Read the model definition and answer for the solid it produces. Units are mm, in the model's axes. Face numbers are marked on the shaded views. A direction names the side the tool comes from. Coordinates: 2 decimals unless noted, no trailing zeros. Order: outer loops, then holes, each group sorted by start corner. A loop starts at its lowest first (then second) coordinate and runs counter-clockwise, first axis right, second up. Notation, with made-up numbers: (-17.5, 41.25) -> (19.5, 41.25) arc R17 ccw to (19.5, 71.25) -> close; hole circle Ø4 at (35, -35). An arc over 180 degrees is marked (long way). Answer in a Markdown table with one row per item.
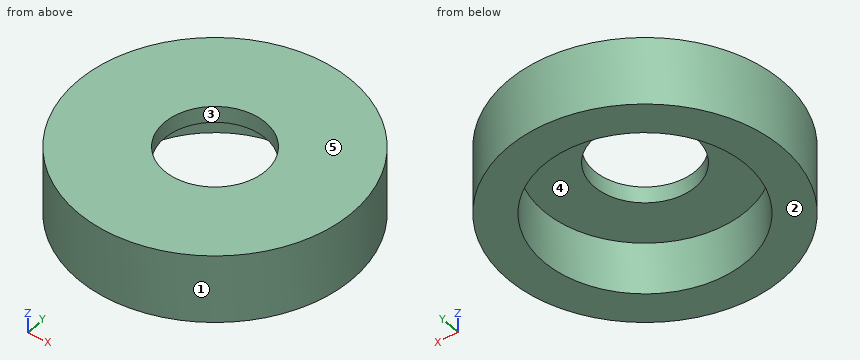
from build123d import *

# Parameters (mm, degrees)
SKETCH_1_R          = 42
EXTRUDE_1_DEPTH     = 21
SKETCH_2_R          = 31
CUT_EXTRUDE_2_DEPTH = 16
SKETCH_3_R          = 15.5
CUT_EXTRUDE_3_DEPTH = 62.514225997


with BuildPart() as part:
    # Эскиз1 → Вытянуть1 (new body)
    with BuildSketch(Plane.XY):
        with Locations(Location((0, 0, 0), (0, 0, 180))):
            Circle(SKETCH_1_R)
    extrude(amount=EXTRUDE_1_DEPTH)

    # Эскиз2 → Вытянуть2 (cut)
    with BuildSketch(Plane(origin=(0, 0, 0), x_dir=(-1, 0, 0), z_dir=(0, 0, -1))):
        Circle(SKETCH_2_R)
    extrude(amount=-CUT_EXTRUDE_2_DEPTH, mode=Mode.SUBTRACT)

    # Эскиз3 → Вытянуть3 (cut, through all)
    with BuildSketch(Plane(origin=(0, 0, 16), x_dir=(-1, 0, 0), z_dir=(0, 0, -1))):
        Circle(SKETCH_3_R)
    extrude(amount=-CUT_EXTRUDE_3_DEPTH, mode=Mode.SUBTRACT)


solid = part.part
Q1. The part is cut by section D-D (y = -17.5). Write down the section's boundary in (x, z).
Outcome:
| item | result |
|---|---|
| outline | (-38.18, 0) -> (-25.59, 0) -> (-25.59, 16) -> (25.59, 16) -> (25.59, 0) -> (38.18, 0) -> (38.18, 21) -> (-38.18, 21) -> close |
Q2. For the marked faces 4 and 5, determine the directions among +Z, -Z, +X, -X, +Y, -Y from which every point of the face is accessible in a straight line to the end or side of a thin tool.
Outcome:
| item | result |
|---|---|
| face 4 | -Z |
| face 5 | +Z, +X, -X, +Y, -Y |
Q3. The part is cut by section C-C (z = 6.75). Write down the section's boundary in (x, y), then the cut area to 3 significant figures.
Outcome:
| item | result |
|---|---|
| outline | circle Ø84 at (0, 0); hole circle Ø62 at (0, 0) |
| area | 2,520 mm² |
Q4. The part is cut by section A-A (x = 0). Write down the section's boundary in (y, z), then the cut area to 3 significant figures.
Outcome:
| item | result |
|---|---|
| outline | (-42, 0) -> (-31, 0) -> (-31, 16) -> (-15.5, 16) -> (-15.5, 21) -> (-42, 21) -> close; (15.5, 16) -> (31, 16) -> (31, 0) -> (42, 0) -> (42, 21) -> (15.5, 21) -> close |
| area | 617 mm² |
Q5. Consider line 1 (Y direction, x = 0, z = 3.5); line 2 (Y direction, x = 0, z = 18.65); line 3 (Z direction, x = 3, y = 28). Determine where each line is inside the solid, lowest interval first.
Outcome:
| item | result |
|---|---|
| line 1 | -42 to -31, 31 to 42 |
| line 2 | -42 to -15.5, 15.5 to 42 |
| line 3 | 16 to 21 |
Q6. For a pull along X with two mould halves and no side action, classify the marked faces 1, 2 and 3 as pulls with the +X half, pulls with the -X half, needs draft (parallel to the pull), parting line crosses it, or undercut.
Outcome:
| item | result |
|---|---|
| face 1 | parting line crosses it |
| face 2 | needs draft |
| face 3 | undercut |
Q7. Given pin 1 (4 mm diameter, centred on x = 16, z = 17, fed in from +Y); pin 2 (12 mm diameter, centred on x = 32.5, y = -7, fed in from -Z); pin 3 (6 mm diameter, centred on x = -32, z = 17.5, fed in from -Y); pin 4 (10 mm diameter, centred on x = -7, z = 11, fed in from +Y), each flat-ended and moving along its own axis, determine where each tip first touches the part or whether it passes through.
Outcome:
| item | result |
|---|---|
| pin 1 | y = 39.6 |
| pin 2 | z = 0 |
| pin 3 | y = -30.38 |
| pin 4 | y = 41.95 |
